from build123d import *

# Parameters (mm, degrees)
EXTRUDE_1_DEPTH             = 6
HOLE_WIZARD_3_D             = 4.5
HOLE_WIZARD_3_CBORE_D       = 8
HOLE_WIZARD_3_CBORE_DEPTH   = 4.6
CUT_EXTRUDE_1_DEPTH         = 1
CUT_EXTRUDE_2_DEPTH         = 1
HOLE_WIZARD_2_D             = 4.5
HOLE_WIZARD_2_CBORE_D       = 7.4
HOLE_WIZARD_2_CBORE_DEPTH   = 4.6
HOLE_WIZARD_3_2_D           = 4.5
HOLE_WIZARD_3_2_CBORE_D     = 7.4
HOLE_WIZARD_3_2_CBORE_DEPTH = 4.6
CUT_EXTRUDE_3_DEPTH         = 86.277077811


with BuildPart() as part:
    # 草图1 → 凸台-拉伸1 (new, symmetric)
    with BuildSketch(Plane(origin=(0, 0, 0), x_dir=(0, 0, -1), z_dir=(1, 0, 0))):
        Polygon((0, 0), (42.02233047, 0), (59.7, -17.67766953), (59.7, -59.7), align=None)
    extrude(amount=EXTRUDE_1_DEPTH, both=True)

    # Hole Wizard 3 (through all)
    with Locations(Plane(origin=(0, 0, 0), x_dir=(1, 0, 0), z_dir=(0, -0.7071067811865477, 0.7071067811865475))):
        with Locations((0, -35.714274837), (0, -48.714274837)):
            CounterBoreHole(HOLE_WIZARD_3_D / 2, HOLE_WIZARD_3_CBORE_D / 2, HOLE_WIZARD_3_CBORE_DEPTH)

    # 草图10 → 切除-拉伸1 (cut)
    with BuildSketch(Plane.ZY.offset(-6)):
        Polygon((-42.02233047, 0), (0, 0), (-10, -10), (-52.02233047, -10), align=None)
    extrude(amount=CUT_EXTRUDE_1_DEPTH, mode=Mode.SUBTRACT)

    # 草图11 → 切除-拉伸2 (cut)
    with BuildSketch(Plane.ZY.offset(6)):
        Polygon((-59.7, -17.67766953), (-59.7, -59.7), (-49.7, -49.7), (-49.7, -7.67766953), align=None)
    extrude(amount=-CUT_EXTRUDE_2_DEPTH, mode=Mode.SUBTRACT)

    # 打孔尺寸根据内六角圆柱头螺钉的类型2 (through all)
    with Locations(Plane.ZY.offset(6)):
        with Locations((-20.011165235, -5), (-32.011165235, -5)):
            CounterBoreHole(HOLE_WIZARD_2_D / 2, HOLE_WIZARD_2_CBORE_D / 2, HOLE_WIZARD_2_CBORE_DEPTH)

    # Hole Wizard 3 2 (through all)
    with Locations(Plane(origin=(6, 0, 0), x_dir=(0, 0, -1), z_dir=(1, 0, 0))):
        with Locations((54.7, -39.688834765), (54.7, -27.688834765)):
            CounterBoreHole(HOLE_WIZARD_3_2_D / 2, HOLE_WIZARD_3_2_CBORE_D / 2, HOLE_WIZARD_3_2_CBORE_DEPTH)

    # 草图16 → 切除-拉伸3 (cut, through all)
    with BuildSketch(Plane(origin=(6, 0, 0), x_dir=(0, 0, -1), z_dir=(1, 0, 0))):
        Polygon((10, -10), (10, 0), (0, 0), align=None)
        Polygon((59.7, -59.7), (59.7, -49.7), (49.7, -49.7), align=None)
    extrude(amount=-CUT_EXTRUDE_3_DEPTH, mode=Mode.SUBTRACT)


solid = part.part
Build history of the part. All positions in model axes, mm. A direction names the side the tool comes from. Round coordinates to 2 decimals unless told otherwise and drop trailing zeros. Write each loop counter-clockwise with the first axis right and the second up, starting at its lowest first coordinate (ties: lowest second). Pieces come first, ordered by that corner, then holes. Notation, with made-up numbers: (77, 40) -> (119, 40) arc R9 cw to (119, 46) -> close; hole circle Ø1 at (35, -30.75). An arc over 180 degrees is marked (long way). Write item = value, one per line.
(1) Tool access for faces 1 (the face through (1.722, -23.219, -29.724)), 2 (the face through (3.73, -26.58, -58.23)), 3 (the face through (5, -5, -26)): list every direction of +Z, -Z, +X, -X, +Y, -Y with a clear straight run to the whole face (end or side of a thin tool).
Answer:
face_1 = none
face_2 = +X
face_3 = +Z, -Z, +X, +Y
(2) Band-saw the part on B-B (y = -44.5). Give the cut face in (x, z), then the cut area to 3 significant figures.
Answer:
outline = (-6, -49.7) -> (-5, -49.7) -> (-5, -59.7) -> (6, -59.7) -> (6, -44.5) -> (-6, -44.5) -> close
area = 172 mm2
(3) Band-saw the part on D-D (z = -32.5). State how many separate pieces and enclosed holes the cut face has, then the cut area to 3 significant figures.
Answer:
separate_pieces = 2
enclosed_holes = 1
area = 289 mm2
(4) Band-saw the part on A-A (x = 0). Give the cut face in (y, z).
Answer:
outline = (-49.7, -59.7) -> (-17.68, -59.7) -> (-15.03, -57.05) -> (-32.78, -39.29) -> (-34.02, -40.53) -> (-37.27, -37.27) -> (-49.7, -49.7) -> close; (-31.62, -31.62) -> (-28.37, -34.87) -> (-29.6, -36.11) -> (-11.84, -53.87) -> (-5.83, -47.86) -> (-23.59, -30.1) -> (-24.83, -31.33) -> (-28.08, -28.08) -> close; (-22.43, -22.43) -> (-19.17, -25.68) -> (-20.41, -26.92) -> (-2.65, -44.67) -> (0, -42.02) -> (0, -10) -> (-10, -10) -> close; hole circle Ø4.5 at (-39.69, -54.7); hole circle Ø4.5 at (-27.69, -54.7); hole circle Ø4.5 at (-5, -32.01); hole circle Ø4.5 at (-5, -20.01)
(5) Two-plate mould, pull along Z, no slides. Class faces 4 (the face through (0, -5, -10)), 5 (the face through (-1.4, -7, -18)), 6 (the face through (1, -33, -59.7)): pulls with the +Z half, pulls with the -Z half, needs draft (parallel to the pull), parting line crosses it, or undercut.
Answer:
face_4 = pulls with the +Z half
face_5 = undercut
face_6 = pulls with the -Z half
(6) Flat gauge pins, fed straight in: pin 1 (1.5 mm diameter, centred on x = -4, z = -45, fed in from +Y); pin 2 (9.5 mm diameter, centred on y = -27.69, z = -54.7, fed in from -X); pin 3 (6 mm diameter, centred on y = -5, z = -32.01, fed in from -X). Where does each tip first touch, or does it go through?
Answer:
pin_1 = -2.23
pin_2 = -5
pin_3 = -1.4
(7) Band-saw the part on C-C (z = -17). Give the cut face in (x, y).
Answer:
outline = (-6, -17) -> (6, -17) -> (6, -10) -> (5, -10) -> (5, 0) -> (-6, 0) -> (-6, -2.85) -> (-1.4, -2.85) -> (-1.4, -7.15) -> (-6, -7.15) -> close
(8) Probe L1, parallel to Y at x = -1.5, z = -54.7; L2, parallel to Z at x = 1.75, y = -30.5; L3, parallel to X at y = -7, z = -29.5. List the from-to ranges inside material, lowest first.
Answer:
L1 = -49.7 to -41.94, -37.44 to -29.94, -25.44 to -16.56
L2 = -59.7 to -57.11, -52.29 to -40.39, -33.31 to -30.5
L3 = -1.4 to 5
